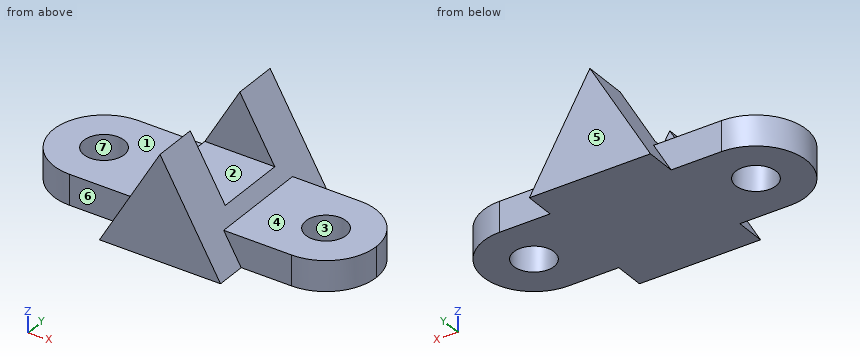
from build123d import *

# Parameters (mm, degrees)
F2_DEPTH = 40
F0_R     = 10
F3_DEPTH = 15
F4_W     = 36
F4_H     = 30
F5_DEPTH = 30


with BuildPart() as f2:
    # F1 (on Front) → F2 (new body, symmetric)
    with BuildSketch(Plane.XZ):
        Polygon((-30, 0), (30, 0), (0, 51.9615242271), align=None)
    extrude(amount=F2_DEPTH, both=True)

    # F0 (on Top) → F3 (join)
    with BuildSketch(Plane.XY):
        with BuildLine():
            ThreePointArc((55, -25), (72.6776695297, -17.6776695297), (80, 0))
            ThreePointArc((80, 0), (72.6776695297, 17.6776695297), (55, 25))
            ThreePointArc((55, 25), (30, 0), (55, -25))
        make_face()
        with Locations((55, 0)):
            Circle(F0_R, mode=Mode.SUBTRACT)
        with BuildLine():
            ThreePointArc((55, -25), (30, 0), (55, 25))
            Line((55, 25), (30, 25))
            Line((30, 25), (0, 25))
            Line((0, 25), (-30, 25))
            Line((-30, 25), (-55, 25))
            ThreePointArc((-55, 25), (-37.3223304703, 17.6776695297), (-30, 0))
            ThreePointArc((-30, 0), (-37.3223304703, -17.6776695297), (-55, -25))
            Line((-55, -25), (-30, -25))
            Line((-30, -25), (0, -25))
            Line((0, -25), (30, -25))
            Line((30, -25), (55, -25))
        make_face()
        with BuildLine():
            ThreePointArc((-30, 0), (-37.3223304703, 17.6776695297), (-55, 25))
            ThreePointArc((-55, 25), (-80, 0), (-55, -25))
            ThreePointArc((-55, -25), (-37.3223304703, -17.6776695297), (-30, 0))
        make_face()
        with Locations((-55, 0)):
            Circle(F0_R, mode=Mode.SUBTRACT)
    extrude(amount=F3_DEPTH)

    # F4 (on Right) → F5 (cut, symmetric)
    with BuildSketch(Plane.YZ):
        with Locations((0, 36.9615242271)):
            Rectangle(F4_W, F4_H)
    extrude(amount=F5_DEPTH, both=True, mode=Mode.SUBTRACT)


solid = f2.part
Here's how the part is built. I have some questions about the finished solid (model axes, mm). Face numbers are marked on the shaded views. A direction names the side the tool comes from. Give positions to 0.01 mm unless a question says otherwise; leave off trailing zeros. Loops run counter-clockwise (first coordinate to the right, second up) from the corner with the lowest first, then second, coordinate; pieces in that order, holes last. Notation, with made-up numbers: (8, 45.25) -> (12, 45.25) arc R23 ccw to (12, 54.25) -> close; hole circle Ø1 at (39.5, 61.5). An arc over 180 degrees is marked (long way). Answer as a JSON object with one key per item and string values. Group by question number.
Item 1: On a 3-axis mill with a long thin cutter (end or side, diameter ignored), from which of +Z, -Z, +X, -X, +Y, -Y can I reach the whole of each face in a straight line? I mean the marked faces 1, 2 and 3. Say none if no direction works.
Item 2: Imagine slicing it at D-D on z = 7. Write out the boundary of the cut face in (x, y), then the cut area to 3 significant figures.
Item 3: Thinking about a two-plate mould opening in Y: for the marked faces 4, 5, 6 and 7, which applies, pulls with the +Y half, pulls with the -Y half, needs draft (parallel to the pull), parting line crosses it, or undercut?
Item 4: Imagine slicing it at B-B on y = -6.5. Write out the boundary of the cut face in (x, z).
Item 5: Imagine slicing it at A-A on z = 27. Write out the boundary of the cut face in (x, y), then the cut area to 3 significant figures.
Item 6: Will these pins go through, and if not, where does the flat tip stop? pin 1 (12 mm diameter, centred on x = -42.5, z = 6, fed in from +Y); pin 2 (4 mm diameter, centred on x = 33.5, z = 13.5, fed in from -Y); pin 3 (25 mm diameter, centred on x = 58, y = 8, fed in from +Z).
Item 7: I need wall thicknesses on L1, parallel to Y at x = 55, z = 6.25; L2, parallel to X at y = -4.5, z = 9; L3, parallel to Z at x = 43, y = -17. Which ranges of each line are inside material? Lowest first, please.
Item 8: Imagine slicing it at C-C on x = -57. Write out the boundary of the cut face in (y, z), then the cut area to 3 significant figures.
Answer list:
{
 "1": {"face 1": "+Z, -X, +Y, -Y", "face 2": "+Z, +X, -X", "face 3": "+Z, -Z"},
 "2": {"outline": "(-55, -25) -> (-25.96, -25) -> (-25.96, -40) -> (25.96, -40) -> (25.96, -25) -> (55, -25) arc R25 ccw to (55, 25) -> (25.96, 25) -> (25.96, 40) -> (-25.96, 40) -> (-25.96, 25) -> (-55, 25) arc R25 ccw to start; hole circle Ø20 at (-55, 0); hole circle Ø20 at (55, 0)", "area": "8,390 mm2"},
 "3": {"face 4": "needs draft", "face 5": "pulls with the +Y half", "face 6": "pulls with the -Y half", "face 7": "undercut"},
 "4": {"outline": "(-79.14, 0) -> (-62.6, 0) -> (-62.6, 15) -> (-79.14, 15) -> close; (-47.4, 0) -> (47.4, 0) -> (47.4, 15) -> (21.34, 15) -> (17.32, 21.96) -> (-17.32, 21.96) -> (-21.34, 15) -> (-47.4, 15) -> close; (62.6, 0) -> (79.14, 0) -> (79.14, 15) -> (62.6, 15) -> close"},
 "5": {"outline": "(-14.41, -40) -> (14.41, -40) -> (14.41, -18) -> (-14.41, -18) -> close; (-14.41, 18) -> (14.41, 18) -> (14.41, 40) -> (-14.41, 40) -> close", "area": "1,270 mm2"},
 "6": {"pin 1": "stops at y = 25", "pin 2": "stops at y = -25", "pin 3": "stops at z = 15"},
 "7": {"L1": "y = -25 to -10, 10 to 25", "L2": "x = -79.59 to -63.93, -46.07 to 46.07, 63.93 to 79.59", "L3": "z = 0 to 15"},
 "8": {"outline": "(-24.92, 0) -> (-9.8, 0) -> (-9.8, 15) -> (-24.92, 15) -> close; (9.8, 0) -> (24.92, 0) -> (24.92, 15) -> (9.8, 15) -> close", "area": "454 mm2"}
}
